The figure shows three views and two pictorial views of one solid part (mm, origin at its lowest corner). Answer the questions. Round coordinates to 2 decimals unless told otherwise and drop trailing zeros. Order: outer loops, then holes, each group sorted by start corner. A loop starts at its lowest first (then second) coordinate and runs counter-clockwise, first axis right, second up. Notation, with made-up numbers: (18.5, 72.5) -> (43.5, 72.5) arc R17 cw to (43.5, 87.5) -> close; hole circle Ø4 at (46, 48.25). An arc over 180 degrees is marked (long way). Return JSON: item names as keys, results as strings. Group by question number.
(1) The part is cut by section B-B (y = 7.5). Count the separate pieces of the cut face and the enclosed holes in it, plus the area to 3 significant figures.
(2) This flat-tipped pin is pushed along its axis until it touches: pin 1 (4.5 mm diameter, centred on x = 109.01, z = 37.01, fed in from -Y). Where does it stop, or does it pass through?
(3) The part is cut by section A-A (x = 88.5). Determine the outline of the cut face in (y, z) (1 decimal), plus the area to 3 significant figures.
(4) The part is cut by section D-D (z = 8). Determine the outline of the cut face in (x, y), plus the area to 3 significant figures.
(5) Consider line 1 (X direction, y = 21.5, z = 45.5) (1 decimal); line 2 (Z direction, x = 88, y = 16.75) (1 decimal); line 3 (X direction, y = 19.5, z = 82) (1 decimal). Determine where each line is inside the solid, lowest interval first. Write a range as [from, to].
(6) The part is cut by section C-C (z = 85.5). Determine the outline of the cut face in (x, y) (1 decimal).
(7) Determine the mould class of the marked faces 1, 2 and 3 for opening direction Y: +Y half, -Y half, draft (parallel to the pull), parting line (faces both ways), or undercut.
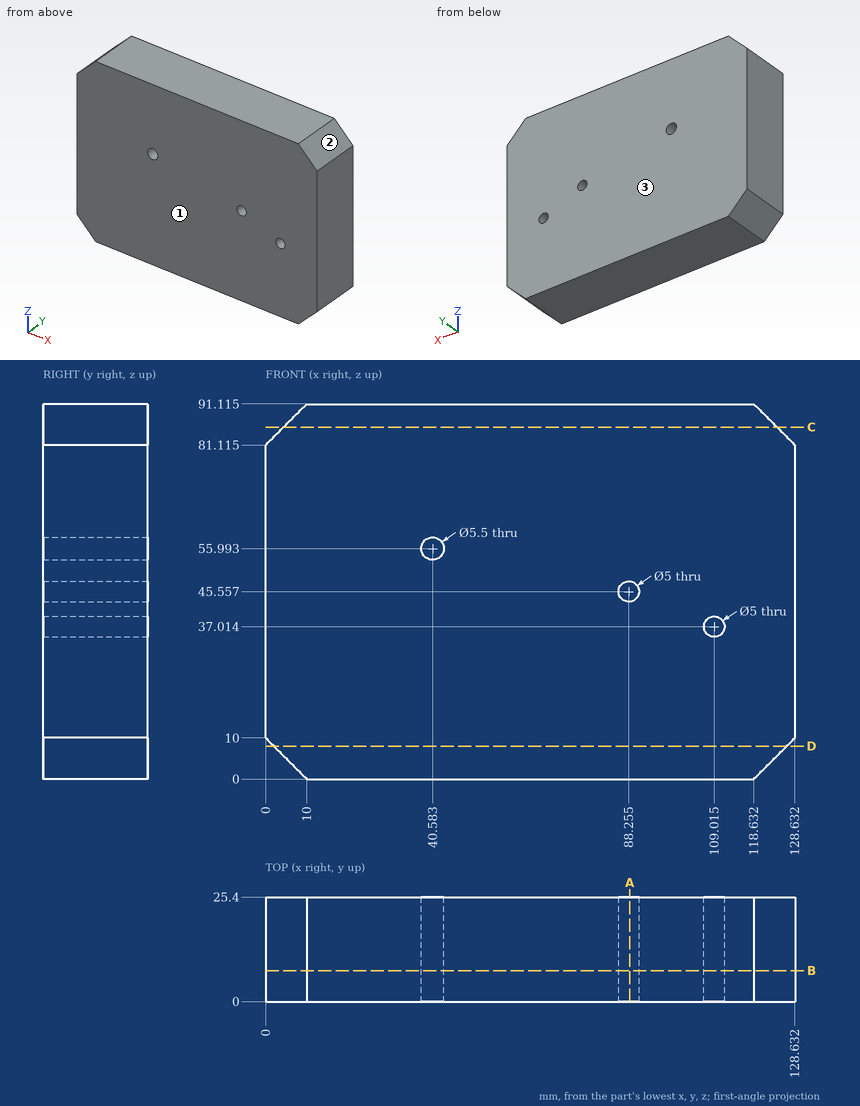
Answer below:
{
 "1": {"separate pieces": "1", "enclosed holes": "3", "area": "11,500 mm²"},
 "2": {"pin 1": "passes through"},
 "3": {"outline": "(0, 0) -> (25.4, 0) -> (25.4, 43.1) -> (0, 43.1) -> close; (0, 48) -> (25.4, 48) -> (25.4, 91.1) -> (0, 91.1) -> close", "area": "2,190 mm²"},
 "4": {"outline": "(2, 0) -> (126.63, 0) -> (126.63, 25.4) -> (2, 25.4) -> close", "area": "3,170 mm²"},
 "5": {"line 1": "x = [0, 85.8], [90.8, 128.6]", "line 2": "z = [0, 43.1], [48, 91.1]", "line 3": "x = [0.9, 127.7]"},
 "6": {"outline": "(4.4, 0) -> (124.2, 0) -> (124.2, 25.4) -> (4.4, 25.4) -> close"},
 "7": {"face 1": "-Y half", "face 2": "draft", "face 3": "+Y half"}
}
